Build history of the part. All positions in model axes, mm. Face numbers are marked on the shaded views. A direction names the side the tool comes from. Give positions to 0.01 mm unless a question says otherwise; leave off trailing zeros. Write each loop counter-clockwise with the first axis right and the second up, starting at its lowest first coordinate (ties: lowest second). Pieces come first, ordered by that corner, then holes. Notation, with made-up numbers: (58, -25.75) - (71, -25.75) arc R27 ccw to (71, -9.75) - close; hole circle Ø1 at (45, 45.25). An arc over 180 degrees is marked (long way). Use one line per item in the form item = value. Start each with the question number.
from build123d import *

# Parameters (mm, degrees)
BOSS_EXTRUDE1_DEPTH = 25.4
SKETCH2_R           = 1.5875
CUT_EXTRUDE1_DEPTH  = 63.965141199
SKETCH3_R           = 9.525
CUT_EXTRUDE2_DEPTH  = 93.653985647
SKETCH4_R           = 1.5875
CUT_EXTRUDE3_DEPTH  = 65.702262374
FILLET1_R           = 2.54


with BuildPart() as part:
    # Sketch1 → Boss-Extrude1 (new body)
    with BuildSketch(Plane.XY):
        with BuildLine():
            Line((-12.3825, 0), (12.3825, 0))
            ThreePointArc((12.3825, 0), (17.145, 4.7625), (21.9075, 0))
            Line((21.9075, 0), (46.99, 0))
            Line((46.99, 0), (46.99, 3.175))
            Line((46.99, 3.175), (36.83, 3.175))
            ThreePointArc((36.83, 3.175), (35.033948776, 3.918948776), (34.29, 5.715))
            Line((34.29, 5.715), (34.29, 36.5125))
            Line((34.29, 36.5125), (-34.29, 36.5125))
            Line((-34.29, 36.5125), (-34.29, 5.715))
            ThreePointArc((-34.29, 5.715), (-35.033948776, 3.918948776), (-36.83, 3.175))
            Line((-36.83, 3.175), (-46.99, 3.175))
            Line((-46.99, 3.175), (-46.99, 0))
            Line((-46.99, 0), (-21.9075, 0))
            ThreePointArc((-21.9075, 0), (-17.145, 4.7625), (-12.3825, 0))
        make_face()
    extrude(amount=BOSS_EXTRUDE1_DEPTH)

    # Sketch2 → Cut-Extrude1 (cut, through all)
    with BuildSketch(Plane(origin=(0, 3.175, 0), x_dir=(1, 0, 0), z_dir=(0, 1, 0))):
        with Locations(Location((40.64, -6.35, 0), (0, 0, 180))):
            Circle(SKETCH2_R)
        with Locations((40.64, -19.05)):
            Circle(SKETCH2_R)
        with Locations((-40.64, -6.35)):
            Circle(SKETCH2_R)
        with Locations(Location((-40.64, -19.05, 0), (0, 0, 180))):
            Circle(SKETCH2_R)
    extrude(amount=-CUT_EXTRUDE1_DEPTH, mode=Mode.SUBTRACT)

    # Sketch3 → Cut-Extrude2 (cut, through all)
    with BuildSketch(Plane(origin=(34.29, 0, 0), x_dir=(0, 0, -1), z_dir=(1, 0, 0))):
        with Locations(Location((-12.7, 23.8125, 0), (0, 0, 90))):
            Circle(SKETCH3_R)
    extrude(amount=-CUT_EXTRUDE2_DEPTH, mode=Mode.SUBTRACT)

    # Sketch4 → Cut-Extrude3 (cut, through all)
    with BuildSketch(Plane.XY.offset(25.4)):
        with Locations((17.145, 23.8125)):
            Circle(SKETCH4_R)
        with Locations((-17.145, 23.8125)):
            Circle(SKETCH4_R)
    extrude(amount=-CUT_EXTRUDE3_DEPTH, mode=Mode.SUBTRACT)

    # Fillet1
    fillet1_edges = [part.edges().sort_by_distance(p)[0] for p in [
        (-41.91, 3.175, 0),
        (-35.033948776, 3.918948776, 0),
        (-34.29, 21.11375, 0),
        (0, 36.5125, 0),
        (41.91, 3.175, 25.4),
        (34.29, 21.11375, 0),
        (35.033948776, 3.918948776, 0),
        (41.91, 3.175, 0),
        (35.033948776, 3.918948776, 25.4),
        (-34.29, 36.5125, 12.7),
        (34.29, 36.5125, 12.7),
        (34.29, 21.11375, 25.4),
        (0, 36.5125, 25.4),
        (-34.29, 21.11375, 25.4),
        (-35.033948776, 3.918948776, 25.4),
        (-41.91, 3.175, 25.4),
    ]]
    fillet(fillet1_edges, radius=FILLET1_R)


solid = part.part
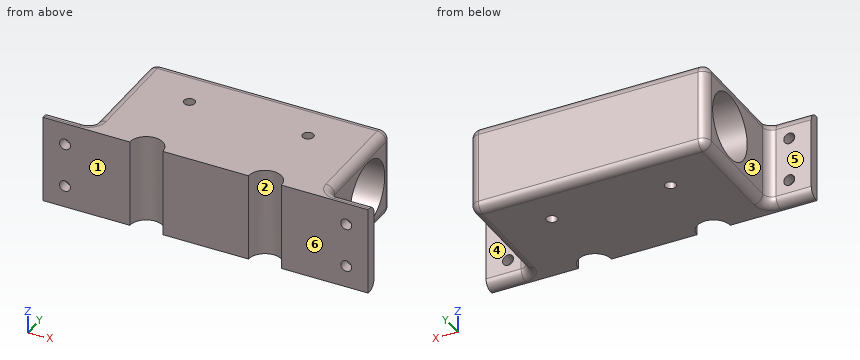
(1) Pin check, flat tips, straight feed: pin 1 Ø3 at (x, z) = (-34, 12) entering from +Y; pin 2 Ø5 at (x, z) = (41.5, 15) entering from +Y (3 decimals); pin 3 Ø6 at (y, z) = (15.5, 13) entering from +X. Stop position of each tip, or through.
(2) Wall check: line 1 (Z direction, x = 40, y = 1); line 2 (X direction, y = 24, z = 23.25); line 3 (Y direction, x = 3, z = 18.25). Give the ranges that are in metal, low to high. Write a range as from..to.
(3) Cut at A-A, the plane x = 40.64. Give the cut face in (y, z) (1 decimal), then the cut area to 3 significant figures.
(4) Which spindle directions (+Z, -Z, +X, -X, +Y, -Y) get a long thin tool onto all of the face, cutting with end or side? Do the marked faces 4, 5 and 6. Say none if no direction does.
(5) Two-plate mould, pull along X, no slides. Class the marked faces 1, 2 and 3: +X half, -X half, draft (parallel to the pull), parting line (faces both ways), or undercut.
(6) Cut at D-D, the plane z = 19.05. State how many separate pieces and enclosed holes the cut face has, then the cut area to 3 significant figures.
(7) Cut at C-C, the plane y = 11.5. Give the cut face in (x, z).
Solution:
q1.pin_1 = 36.4
q1.pin_2 = 3.175
q1.pin_3 = 34.29
q2.line_1 = 0.03..4.9, 7.8..17.6, 20.5..25.37
q2.line_2 = -34.26..-18.72, -15.57..15.57, 18.72..34.26
q2.line_3 = 0..16.07, 31.55..36.51
q3.outline = (0, 0) - (0.6, 0) arc R2.5 ccw to (3.2, 2.5) - (3.2, 4.8) - (0, 4.8) - close; (0, 7.9) - (3.2, 7.9) - (3.2, 17.5) - (0, 17.5) - close; (0, 20.6) - (3.2, 20.6) - (3.2, 22.9) arc R2.5 ccw to (0.6, 25.4) - (0, 25.4) - close
q3.area = 57.7 mm2
q4.face_4 = +Z, -Z, +X, +Y
q4.face_5 = +Z, -Z, -X, +Y
q4.face_6 = +Z, -Z, +X, -X, -Y
q5.face_1 = draft
q5.face_2 = undercut
q5.face_3 = -X half
q6.separate_pieces = 4
q6.enclosed_holes = 0
q6.area = 1,520 mm2
q7.outline = (-34.29, 2.54) arc R2.54 ccw to (-31.75, 0) - (31.75, 0) arc R2.54 ccw to (34.29, 2.54) - (34.29, 22.86) arc R2.54 ccw to (31.75, 25.4) - (-31.75, 25.4) arc R2.54 ccw to (-34.29, 22.86) - close
